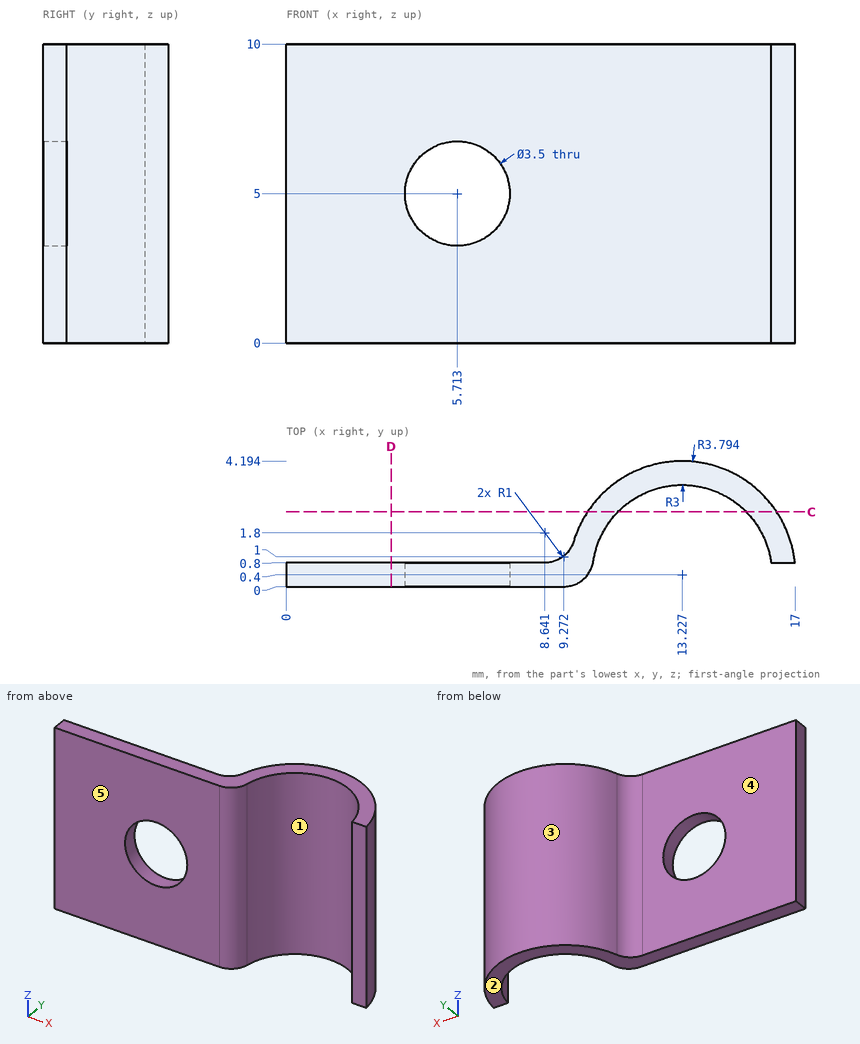
Design review of the part shown in the three views and the two pictorial views. Dimensions are in mm from the part's minimum x, y and z. A direction names the side the tool comes from. Coordinates: 2 decimals unless noted, no trailing zeros. Order: outer loops, then holes, each group sorted by start corner. A loop starts at its lowest first (then second) coordinate and runs counter-clockwise, first axis right, second up.
1) For the marked faces 4 and 5, list the 3-axis set-ups (+Z, -Z, +X, -X, +Y, -Y) from which the entire face can be reached by the end or side of a thin tool; tool diameter is ignored.
2) Wall thickness on line 1 along Y through (x, z) = (7.5, 9); line 2 along X through (y, z) = (0.4, 5) (1 decimal); line 3 along X through (y, z) = (2.8, 8) (1 decimal): over which ranges is each line inside the solid? List them lowest first.
3) Mouldability with a two-part tool opening along X and no side actions: class the marked faces 1, 2 and 3 as +X half, -X half, draft (parallel to the pull), parting line (faces both ways), or undercut.
4) Clearance check with flat-ended pins moving along their axes: pin 1 (2.5 mm diameter, centred on x = 4, z = 3, fed in from +Y); pin 2 (0.9 mm diameter, centred on x = 16.5, z = 7.5, fed in from -Y); pin 3 (4.5 mm diameter, centred on x = 5.71, z = 5, fed in from -Y). State where each tip first meets the part, or that it passes through.
5) Take a section at D-D, the plane x = 3.5. Give the boundary of the cut face in (y, z).
6) Take a section at C-C, the plane y = 2.5. Give the boundary of the cut face in (x, z) (1 decimal).
Returned:
1. face 4: +Z, -Z, -X, +Y
1. face 5: +Z, -Z, +X, -X, -Y
2. line 1: y = 0 to 0.8
2. line 2: x = 0 to 4, 7.5 to 10.1
2. line 3: x = 10.3 to 11.4, 15 to 16.2
3. face 1: undercut
3. face 2: draft
3. face 3: parting line
4. pin 1: stops at y = 0.8
4. pin 2: stops at y = 0.8
4. pin 3: stops at y = 0
5. outline: (0, 0) - (0.8, 0) - (0.8, 10) - (0, 10) - close
6. outline: (10.1, 0) - (11.1, 0) - (11.1, 10) - (10.1, 10) - close; (15.4, 0) - (16.4, 0) - (16.4, 10) - (15.4, 10) - close
